Could you check a few things on this drawing? It's one solid part, dimensions in mm from its lowest x, y, z. A direction names the side the tool comes from. Round coordinates to 2 decimals unless told otherwise and drop trailing zeros. Loops run counter-clockwise (first coordinate to the right, second up) from the corner with the lowest first, then second, coordinate; pieces in that order, holes last. Notation, with made-up numbers: M 11,-15 L 29,-15 A20 cw 29,-10 Z; hole C -11,-35.5 d6. An arc over 180 degrees is marked long. Answer as CSV lines item,"result".
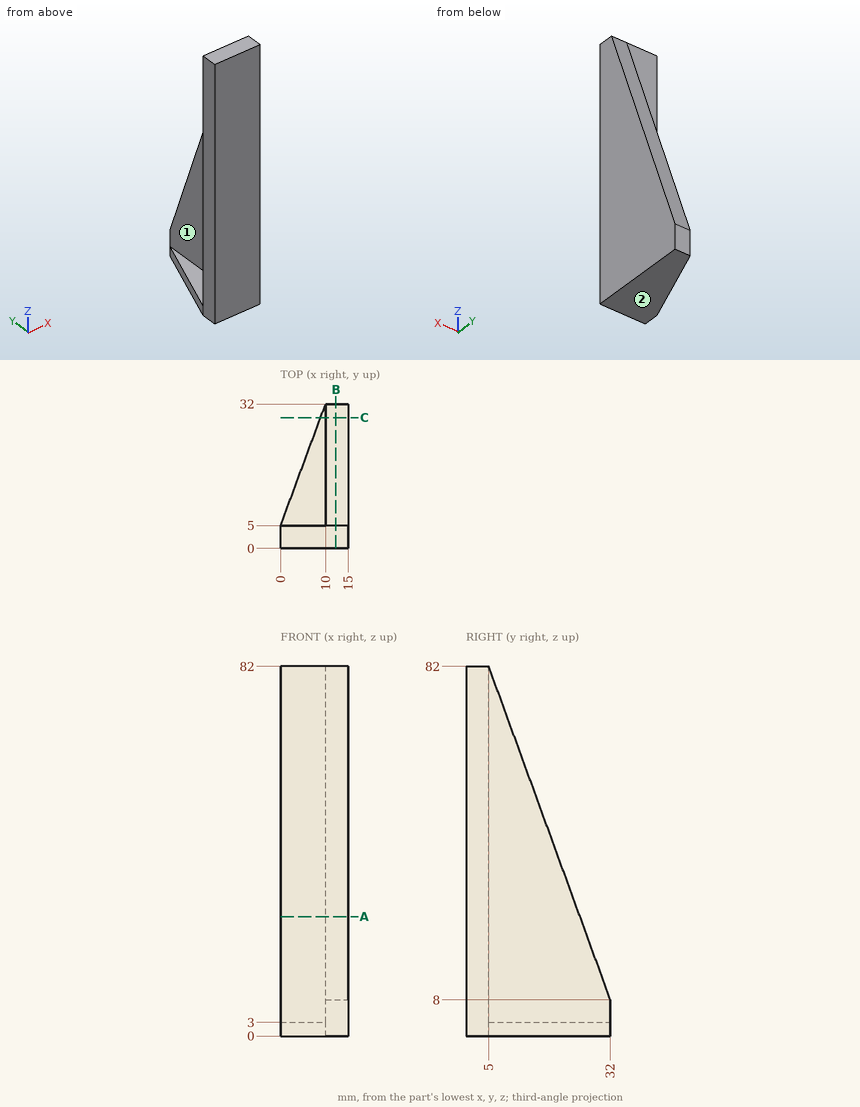
Item 1: If we section it at B-B on x = 12.25: Write out the boundary of the cut face in (y, z), then the cut area to 4 significant figures.
Output:
outline,"M 0,0 L 32,0 L 32,8 L 5,82 L 0,82 Z"
area,"1,625 mm2"
Item 2: Will these pins go through, and if not, where does the flat tip stop? pin 1 (2 mm diameter, centred on x = 3.5, z = 27.5, fed in from +Y); pin 2 (3 mm diameter, centred on x = 5.5, y = 19, fed in from +Z); pin 3 (6 mm diameter, centred on y = 10, z = 69.5, fed in from -X).
Output:
pin 1,"stops at y = 5"
pin 2,"stops at z = 3"
pin 3,"stops at x = 10"
Item 3: If we section it at C-C on y = 29: Write out the boundary of the cut face in (x, z).
Output:
outline,"M 8.89,0 L 15,0 L 15,16.22 L 10,16.22 L 10,3 L 8.89,3 Z"
Item 4: If we section it at A-A on z = 26.5: Write out the boundary of the cut face in (x, y).
Output:
outline,"M 0,0 L 15,0 L 15,25.25 L 10,25.25 L 10,5 L 0,5 Z"
Item 5: If I drill on line 1 along Y through (x, z) = (8.75, 49); line 2 along Z through (x, y) = (8.75, 19); line 3 along X through (y, z) = (10, 7), over which ranges is the centre line in solid material (lowest first)? Write a range as from..to.
Output:
line 1,"y = 0..5"
line 2,"z = 0..3"
line 3,"x = 10..15"
Item 6: On a 3-axis mill with a long thin cutter (end or side, diameter ignored), from which of +Z, -Z, +X, -X, +Y, -Y can I reach the whole of each face in a straight line? I mean the marked faces 1 and 2. Say none if no direction works.
Output:
face 1,"+Z, -X, +Y"
face 2,"-Z, +X, -X, +Y, -Y"
